Read the model definition and answer for the solid it produces. Units are mm, in the model's axes. Face numbers are marked on the shaded views. A direction names the side the tool comes from. Coordinates: 2 decimals unless noted, no trailing zeros. Order: outer loops, then holes, each group sorted by start corner. A loop starts at its lowest first (then second) coordinate and runs counter-clockwise, first axis right, second up.
```python
from build123d import *

# Parameters (mm, degrees)
SKETCH_1_R          = 2.5
EXTRUDE_1_DEPTH     = 8
FILLET_8_R          = 1
SKETCH_2_R          = 2.5
EXTRUDE_2_DEPTH     = 2.5
FILLET_7_R          = 2.5
SKETCH_3_R          = 2.5
EXTRUDE_3_DEPTH     = 8.7
FILLET_4_R          = 2.5
FILLET_5_R          = 1
FILLET_6_R          = 1
SKETCH_4_R          = 2.5
CUT_EXTRUDE_1_DEPTH = 3
SKETCH_5_R          = 2.5
CUT_EXTRUDE_2_DEPTH = 1.5
SKETCH_7_R          = 1.5
EXTRUDE_4_DEPTH     = 1.5
FILLET_9_R          = 1


with BuildPart() as part:
    # 스케치1 → 보스-돌출1 (new body)
    with BuildSketch(Plane.XY):
        with BuildLine():
            Line((-11, 0.25), (-5.25, 6))
            Line((-5.25, 6), (10.645895628, 6))
            ThreePointArc((10.645895628, 6), (15.322947814, 5.028470802), (20, 6))
            Line((20, 6), (20, -2))
            Line((20, -2), (14, -2))
            ThreePointArc((14, -2), (6.928932188, -4.928932188), (4, -12))
            Line((4, -12), (4, -35))
            ThreePointArc((4, -35), (-3.221957743, -50.400925483), (4.620254931, -65.495456935))
            ThreePointArc((4.620254931, -65.495456935), (5.101546116, -66.864569331), (4.000000416, -67.809401077))
            ThreePointArc((4.000000416, -67.809401077), (-10.595076269, -56.067028756), (-14.785374908, -37.809401077))
            Line((-14.785374908, -37.809401077), (-33, -37.809401077))
            Line((-33, -37.809401077), (-33, -34.809401077))
            Line((-33, -34.809401077), (-8.5, -33.675426481))
            Line((-8.5, -33.675426481), (-8.5, -26.675426481))
            Line((-8.5, -26.675426481), (-3, -24.673590192))
            Line((-3, -24.673590192), (-3, -3.673590192))
            Line((-3, -3.673590192), (-11, -1.493890685))
            Line((-11, -1.493890685), (-11, 0.25))
        make_face()
        Circle(SKETCH_1_R, mode=Mode.SUBTRACT)
    extrude(amount=EXTRUDE_1_DEPTH)

    # 필렛8
    fillet_8_edges = [part.edges().sort_by_distance(p)[0] for p in [
        (4, -35, 4),
        (-14.785374908, -37.809401077, 4),
        (-8.5, -33.675426481, 4),
    ]]
    fillet(fillet_8_edges, radius=FILLET_8_R)

    # 스케치2 → 보스-돌출2 (add)
    with BuildSketch(Plane.ZY.offset(3)):
        with Locations(Location((4, -9.673590192, 0), (0, 0, 90))):
            Circle(SKETCH_2_R)
    extrude(amount=EXTRUDE_2_DEPTH)

    # 필렛7
    fillet_7_edges = [part.edges().sort_by_distance(p)[0] for p in [
        (-5.5, -12.173590192, 4),
    ]]
    fillet(fillet_7_edges, radius=FILLET_7_R - 0.0001)  # a hair under: the kernel refuses the full size

    # 스케치3 → 보스-돌출3 (add)
    with BuildSketch(Plane(origin=(7.579005696, -20.823147011, 0), x_dir=(0.9396926207859105, 0.34202014332566305, 0), z_dir=(-0.34202014332566305, 0.9396926207859105, 0))):
        with Locations((-14.184431591, -4)):
            Circle(SKETCH_3_R)
    extrude(amount=EXTRUDE_3_DEPTH)

    # 필렛4
    fillet_4_edges = [part.edges().sort_by_distance(p)[0] for p in [
        (-11.074806799, -18.354232894, 4),
    ]]
    fillet(fillet_4_edges, radius=FILLET_4_R)

    # 필렛5
    fillet_5_edges = [part.edges().sort_by_distance(p)[0] for p in [
        (20, 6, 4),
    ]]
    fillet(fillet_5_edges, radius=FILLET_5_R)

    # 필렛6
    fillet_6_edges = [part.edges().sort_by_distance(p)[0] for p in [
        (-11, 0.25, 4),
        (-5.25, 6, 4),
    ]]
    fillet(fillet_6_edges, radius=FILLET_6_R)

    # 스케치4 → 컷-돌출1 (cut)
    with BuildSketch(Plane.XZ.offset(2)):
        with Locations(Location((16.726046575, 4, 0), (0, 0, 270))):
            Circle(SKETCH_4_R)
    extrude(amount=-CUT_EXTRUDE_1_DEPTH, mode=Mode.SUBTRACT)

    # 스케치5 → 컷-돌출2 (cut)
    with BuildSketch(Plane(origin=(1.537153943, -33.210860048, 0), x_dir=(0.9989305822499971, 0.046235179740992706, 0), z_dir=(-0.046235179740992706, 0.9989305822499971, 0))):
        with Locations(Location((-30.57412813, -4, 0), (0, 0, 180))):
            Circle(SKETCH_5_R)
    extrude(amount=-CUT_EXTRUDE_2_DEPTH, mode=Mode.SUBTRACT)

    # 스케치7 → 보스-돌출4 (add)
    with BuildSketch(Plane(origin=(1.606506713, -34.709255922, 0), x_dir=(0.9989305822499971, 0.04623517974099271, 0), z_dir=(-0.04623517974099271, 0.9989305822499971, 0))):
        with Locations(Location((-30.57412813, -4, 0), (0, 0, 180))):
            Circle(SKETCH_7_R)
    extrude(amount=EXTRUDE_4_DEPTH)

    # 필렛9
    fillet_9_edges = [part.edges().sort_by_distance(p)[0] for p in [
        (-27.505881798, -34.555107588, 4),
    ]]
    fillet(fillet_9_edges, radius=FILLET_9_R)


solid = part.part
```
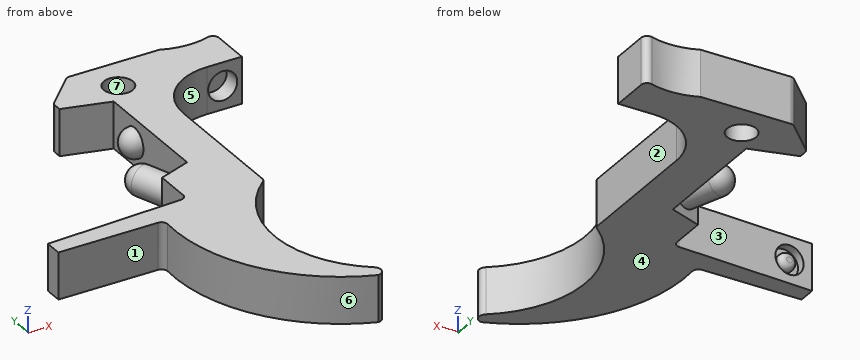
1) Flat-ended cylindrical pins translate along their axes: pin 1 Ø3 at (y, z) = (-28.5, 4.5) entering from -X; pin 2 Ø1.5 at (x, z) = (-20.5, 6) entering from +Y; pin 3 Ø2.5 at (y, z) = (-26, 5.5) entering from +X; pin 4 Ø3 at (x, y) = (0, 0) entering from -Z. Find the tip coordinate at first contact, or state that the pin passes through.
A:
pin 1: stops at x = -8.5
pin 2: stops at y = -34.2
pin 3: stops at x = 4
pin 4: passes through
2) A cutting plane is placed at B-B, the plane y = -57. Determine the outline of the cut face in (x, z).
A:
outline: (-9.99, 0) - (-1.91, 0) - (-1.91, 8) - (-9.99, 8) - close
3) Straight lines are drawn through the part: line 1 (X direction, y = -0.45, z = 4); line 2 (Y direction, x = 1.5, z = 6.25); line 3 (X direction, y = -30, z = 1.75). For each, find the intervals that lie inside material, in ascending order.
A:
line 1: x = -11 to -2.46, 2.46 to 14.23, 19.23 to 20
line 2: y = -66.78 to -62.63, -37.39 to -2, 2 to 6
line 3: x = -8.5 to 4
4) A cutting plane is placed at A-A, the plane x = 0. Determine the outline of the cut face in (y, z), and give its area (3 significant figures).
A:
outline: (-66.02, 0) - (-60.66, 0) - (-60.66, 8) - (-66.02, 8) - close; (-39.36, 0) - (-2.5, 0) - (-2.5, 8) - (-39.36, 8) - close; (2.5, 0) - (6, 0) - (6, 8) - (2.5, 8) - close
area: 366 mm2
5) Which of the six approach directions +Z, -Z, +X, -X, +Y, -Y give full straight-line access (tool end or side, diameter ignored) to the marked faces 1, 2 and 3?
A:
face 1: +Z, -Z, -X, -Y
face 2: +Z, -Z, +X
face 3: +Z, -Z, -X
6) A cutting plane is placed at C-C, the plane x = -18.5. Determine the outline of the cut face in (y, z).
A:
outline: (-37.81, 0) - (-34.14, 0) - (-34.14, 8) - (-37.81, 8) - close
7) Determine the mould class of the marked faces 4, 5, 6 and 7 for opening direction X: pulls with the +X half, pulls with the -X half, needs draft (parallel to the pull), parting line crosses it, or undercut.
A:
face 4: needs draft
face 5: pulls with the +X half
face 6: pulls with the -X half
face 7: undercut
